Autodesk Inventor part; units mm, degrees
ref_plane "YZ Plane" through (0, 0, 0) normal (1, 0, 0) x (0, 1, 0)
ref_plane "XZ Plane" through (0, 0, 0) normal (0, 1, 0) x (-1, 0, 0)
ref_plane "XY Plane" through (0, 0, 0) normal (0, 0, 1) x (1, 0, 0)
sketch "Skizze1" plane through (0, 0, 0) normal (1, 0, 0) x (0, 1, 0)
  line L0 (20, 20) -> (-20, 20)
  line L1 (-20, 20) -> (-20, -20)
  line L2 (-20, -20) -> (20, -20)
  line L3 (20, -20) -> (20, 20)
  line L4 (20, 20) -> (-20, -20) construction
  line L5 (-20, 20) -> (20, -20) construction
  point P0 (0, 0)
  dimension "d0" = 40
  dimension "d1" = 40
extrude "Extrusion1" add sketch "Skizze1" along normal blind 25
sketch "Skizze2" plane through (25, 0, 0) normal (1, 0, 0) x (0, 0, -1)
  line L0 (-25, 25) -> (25, 25)
  line L1 (25, 25) -> (25, -25)
  line L2 (25, -25) -> (-25, -25)
  line L3 (-25, -25) -> (-25, 25)
  line L4 (-25, 25) -> (25, -25) construction
  line L5 (25, 25) -> (-25, -25) construction
  point P0 (0, 0)
  dimension "d4" = 50
  dimension "d5" = 50
extrude "Extrusion2" add sketch "Skizze2" against normal blind 12.5
sketch "Skizze3" plane through (25, 0, 0) normal (1, 0, 0) x (0, 0, -1)
  point P0 (0, 0)
  point P1 (21, -21)
  point P2 (-21, -21)
  point P3 (-21, 21)
  point P4 (21, 21)
  point P5 (16, -16)
  point P6 (-16, -16)
  point P7 (-16, 16)
  point P8 (16, 16)
hole "Bohrung1" at (25, -21, -21) at (25, -21, 21) at (25, 21, 21) at (25, 21, -21) at (25, -16, -16) at (25, -16, 16) at (25, 16, 16) at (25, 16, -16) direction (-1, 0, 0) diameter 2.8 depth 230
sketch "Skizze4" plane through (25, 0, 0) normal (1, 0, 0) x (0, 0, -1)
  circle A0 centre (-16, 16) radius 1.4
  circle A1 centre (16, -16) radius 1.4
  circle A2 centre (-21, 21) radius 1.4
  circle A3 centre (21, -21) radius 1.4
  circle A4 centre (-21, -21) radius 1.4
  circle A5 centre (21, 21) radius 1.4
  circle A6 centre (-16, -16) radius 1.4
  circle A7 centre (16, 16) radius 1.4
  line L0 (-25, -25) -> (25, -25)
  line L1 (25, -25) -> (25, 25)
  line L2 (25, 25) -> (-25, 25)
  line L3 (-25, 25) -> (-25, -25)
  circle A8 centre (-16, 16) radius 1.4
  circle A9 centre (16, 16) radius 1.4
  circle A10 centre (16, -16) radius 1.4
  point P0 (0, 0)
hole "Bohrung2" at (25, 16, 16) at (25, 16, -16) at (25, -16, -16) at (25, -16, 16) direction (-1, 0, 0) diameter 4.2 depth 230 counterbore diameter 8 counterbore depth 4
properties part number "OCT_SpiegelAdapter_MovingSt."
Design review of the part built by this model. Coordinates are the model's own, in mm. A direction names the side the tool comes from. Give positions to 0.01 mm unless a question says otherwise; leave off trailing zeros. Order: outer loops, then holes, each group sorted by start corner. A loop starts at its lowest first (then second) coordinate and runs counter-clockwise, first axis right, second up.
1. For pin 1 Ø4 at (x, z) = (9, 2.5) entering from +Y; pin 2 Ø6 at (x, z) = (3, -2) entering from -Y; pin 3 Ø2.5 at (y, z) = (-14.5, -16) entering from +X, all flat-tipped, find the tip position at first contact; note any pin that passes through.
Solution:
pin 1: stops at y = 20
pin 2: stops at y = -20
pin 3: stops at x = 21
2. Add section D-D, the plane x = 16.25. State how many separate pieces and enclosed holes the cut face has, then the cut area to 3 significant figures.
Solution:
separate pieces: 1
enclosed holes: 8
area: 2,420 mm2
3. To check wall thickness, follow L1, parallel to Y at x = 17.25, z = 21; L2, parallel to Z at x = 23.8, y = 16; L3, parallel to Y at x = 14, z = 16. State the ranges of each line that lie inside material, in increasing order.
Solution:
L1: y = -25 to -22.4, -19.6 to 19.6, 22.4 to 25
L2: z = -25 to -20, -12 to 12, 20 to 25
L3: y = -25 to -18.1, -13.9 to 13.9, 18.1 to 25
4. Tool access review of faces 5 (the flat face through (6, 0, -20)), 6 (the flat face through (6, 0, 20)), 7 (the cylindrical face through (22.97, -18.7, 18.95)), 8 (the flat face through (19, 0, -25)): name each direction out of +Z, -Z, +X, -X, +Y, -Y from which nothing blocks a thin tool from reaching the whole face with its end or side.
Solution:
face 5: -Z, -X, +Y, -Y
face 6: +Z, -X, +Y, -Y
face 7: +X
face 8: -Z, +X, -X, +Y, -Y
5. Mouldability with a two-part tool opening along Y and no side actions: class faces 1 (the cylindrical face through (10.353, -18.082, -15.727)), 2 (the flat face through (25, 0, 0)), 3 (the flat face through (19, 25, 0)), 4 (the cylindrical face through (18.66, -19.76, 20.35)) as +Y half, -Y half, draft (parallel to the pull), parting line (faces both ways), or undercut.
Solution:
face 1: undercut
face 2: draft
face 3: +Y half
face 4: undercut
6. Add section C-C, the plane x = 9. State the section outline as (y, z) points.
Solution:
outline: (-20, -20) - (20, -20) - (20, 20) - (-20, 20) - close; hole circle Ø4.2 at (-16, -16); hole circle Ø4.2 at (-16, 16); hole circle Ø4.2 at (16, -16); hole circle Ø4.2 at (16, 16)
7. Add section A-A, the plane y = 16. State the section outline as (x, z) points.
Solution:
outline: (0, -20) - (12.5, -20) - (12.5, -25) - (25, -25) - (25, -20) - (21, -20) - (21, -18.1) - (0, -18.1) - close; (0, -13.9) - (21, -13.9) - (21, -12) - (25, -12) - (25, 12) - (21, 12) - (21, 13.9) - (0, 13.9) - close; (0, 18.1) - (21, 18.1) - (21, 20) - (25, 20) - (25, 25) - (12.5, 25) - (12.5, 20) - (0, 20) - close
